Here's how the part is built. I have some questions about the finished solid (model axes, mm). Face numbers are marked on the shaded views. A direction names the side the tool comes from. Give positions to 0.01 mm unless a question says otherwise; leave off trailing zeros. Write each loop counter-clockwise with the first axis right and the second up, starting at its lowest first coordinate (ties: lowest second). Pieces come first, ordered by that corner, then holes. Notation, with made-up numbers: (56.5, 2) - (63.5, 2) arc R36 ccw to (63.5, 41) - close; hole circle Ø4 at (62.25, 27.25). An arc over 180 degrees is marked (long way). Use a Markdown table: item, result.
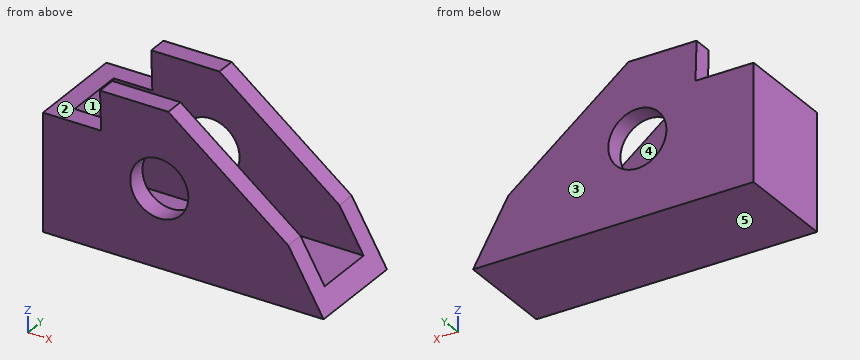
```python
from build123d import *

# Parameters (mm, degrees)
F0_R     = 9.525
F1_DEPTH = 33.02
F2_W     = 12.3416540065
F2_H     = 20.32
F2_W_2   = 22.352
F2_W_3   = 50.9043459935
F3_DEPTH = 44.45


with BuildPart() as f1:
    # F0 (on Front) → F1 (new body)
    with BuildSketch(Plane.XZ):
        Polygon((2.9436540065, 25.3949434087), (-19.4083459935, 25.3949434087), (-19.05, 12.7), (-38.1, 12.7), (-38.1, -25.4), (53.848, -25.4), (42.2530133757, -5.3168940537), align=None)
        Circle(F0_R, mode=Mode.SUBTRACT)
    extrude(amount=F1_DEPTH)

    # F2 (on face) → F3 (cut)
    with BuildSketch(Plane.XY.offset(25.3949434087)):
        with Locations((-25.5791729967, -16.51)):
            Rectangle(F2_W, F2_H)
        with Locations((-8.2323459935, -16.51)):
            Rectangle(F2_W_2, F2_H)
        with Locations((28.3958270033, -16.51)):
            Rectangle(F2_W_3, F2_H)
    extrude(amount=-F3_DEPTH, mode=Mode.SUBTRACT)


solid = f1.part
```
Item 1: If we section it at D-D, the plane y = -24: Write out the boundary of the cut face in (x, z), plus the area to 3 significant figures.
Values:
| item | result |
|---|---|
| outline | (-38.1, -25.4) - (53.85, -25.4) - (50.18, -19.06) - (-31.75, -19.06) - (-31.75, 12.7) - (-38.1, 12.7) - close |
| area | 773 mm2 |
Item 2: If we section it at C-C, the plane z = 0: Write out the boundary of the cut face in (x, y) (3 decimals).
Values:
| item | result |
|---|---|
| outline | (-38.1, -33.02) - (-9.525, -33.02) - (-9.525, -26.67) - (-31.75, -26.67) - (-31.75, -6.35) - (-9.525, -6.35) - (-9.525, 0) - (-38.1, 0) - close; (9.525, -33.02) - (35.448, -33.02) - (35.448, -26.67) - (9.525, -26.67) - close; (9.525, -6.35) - (35.448, -6.35) - (35.448, 0) - (9.525, 0) - close |
Item 3: I need wall thicknesses on line 1 along Y through (x, z) = (22, 5); line 2 along Z through (x, y) = (0, -1) (3 decimals); line 3 along X through (y, z) = (-9.5, -10). Which ranges of each line are inside material? Lowest first, please. Write a range as [from, to].
Values:
| item | result |
|---|---|
| line 1 | y = [-33.02, -26.67], [-6.35, 0] |
| line 2 | z = [-25.4, -9.525], [9.525, 25.395] |
| line 3 | x = [-38.1, -31.75] |
Item 4: For the marked faces 4 and 5, which set-ups out of +Z, -Z, +X, -X, +Y, -Y let a thin tool reach every point of the face, with its end or its side?
Values:
| item | result |
|---|---|
| face 4 | +Z, +X |
| face 5 | -Z, +X, -X, +Y, -Y |
Item 5: Will these pins go through, and if not, where does the flat tip stop? pin 1 Ø1 at (x, y) = (43.5, -5) entering from +Z; pin 2 Ø1 at (y, z) = (-17.5, 14) entering from +X; pin 3 Ø10 at (x, y) = (15.5, -17.5) entering from +Z; pin 4 Ø4 at (x, y) = (15.5, -7) entering from +Z.
Values:
| item | result |
|---|---|
| pin 1 | stops at z = -6.61 |
| pin 2 | passes through |
| pin 3 | stops at z = -19.06 |
| pin 4 | stops at z = 17.06 |
Item 6: If we section it at B-B, the plane y = -4.5: Write out the boundary of the cut face in (x, z) (3 decimals).
Values:
| item | result |
|---|---|
| outline | (-38.1, -25.4) - (53.848, -25.4) - (42.253, -5.317) - (2.944, 25.395) - (-19.408, 25.395) - (-19.05, 12.7) - (-38.1, 12.7) - close; hole circle Ø19.05 at (0, 0) |
Item 7: If we section it at A-A, the plane x = 0: Write out the boundary of the cut face in (y, z) (3 decimals), plus the area to 3 significant figures.
Values:
| item | result |
|---|---|
| outline | (-33.02, -25.4) - (0, -25.4) - (0, -9.525) - (-6.35, -9.525) - (-6.35, -19.055) - (-26.67, -19.055) - (-26.67, -9.525) - (-33.02, -9.525) - close; (-33.02, 9.525) - (-26.67, 9.525) - (-26.67, 25.395) - (-33.02, 25.395) - close; (-6.35, 9.525) - (0, 9.525) - (0, 25.395) - (-6.35, 25.395) - close |
| area | 532 mm2 |
Item 8: Thinking about a two-plate mould opening in Y: for the marked faces 1, 2 and 3, which applies, +Y half, -Y half, draft (parallel to the pull), parting line (faces both ways), or undercut?
Values:
| item | result |
|---|---|
| face 1 | undercut |
| face 2 | draft |
| face 3 | +Y half |
